```python
from build123d import *

# Parameters (mm, degrees)
F2_DEPTH = 2.5
F3_R     = 3
F4_R     = 20


with BuildPart() as f2:
    # F1 (on Top) → F2 (new body)
    with BuildSketch(Plane.XY):
        with BuildLine():
            Line((2.488848, -10.5), (-2.488848, -10.5))
            Line((-2.488848, -10.5), (-2.488848, -9.168186))
            ThreePointArc((-2.488848, -9.168186), (-4.247392, -2.645334), (-8.899342, 2.253587))
            Line((-8.899342, 2.253587), (-8.899342, 6.253587))
            Line((-8.899342, 6.253587), (-15, 6.253587))
            Line((-15, 6.253587), (-10, -23.746413))
            Line((-10, -23.746413), (-10, -83.746413))
            ThreePointArc((-10, -83.746413), (0, -93.746413), (10, -83.746413))
            Line((10, -83.746413), (10, -23.746413))
            Line((10, -23.746413), (15, 6.253587))
            Line((15, 6.253587), (8.899342, 6.253587))
            Line((8.899342, 6.253587), (8.899342, 2.253587))
            ThreePointArc((8.899342, 2.253587), (4.247392, -2.645334), (2.488848, -9.168186))
            Line((2.488848, -9.168186), (2.488848, -10.5))
        make_face()
    extrude(amount=F2_DEPTH)

    # F3
    f3_edges = [f2.edges().sort_by_distance(p)[0] for p in [
        (-15, 6.253587, 1.25),
        (15, 6.253587, 1.25),
    ]]
    fillet(f3_edges, radius=F3_R)

    # F4
    f4_edges = [f2.edges().sort_by_distance(p)[0] for p in [
        (-10, -23.746413, 1.25),
        (10, -23.746413, 1.25),
    ]]
    fillet(f4_edges, radius=F4_R)


solid = f2.part
```
Verification items for the finished model (mm, model axes). A direction names the side the tool comes from. Coordinates: 2 decimals unless noted, no trailing zeros. Order: outer loops, then holes, each group sorted by start corner. A loop starts at its lowest first (then second) coordinate and runs counter-clockwise, first axis right, second up. Notation, with made-up numbers: (54.25, -28) -> (94.25, -28) arc R22 ccw to (94.25, 10) -> close; hole circle Ø10 at (0.25, 2). An arc over 180 degrees is marked (long way). Answer as CSV lines item,"result". Start each with the question number.
1) Material ranges on L1, parallel to X at y = -59.5, z = 2.35; L2, parallel to Y at x = 0, z = 0.25; L3, parallel to Y at x = 8.5, z = 0.8, recorded low to high. Write a range as [from, to].
2) Set-up check for faces 1 (the face through (-10, 6.254, 1)), 2 (the face through (10, -55, 1)), 3 (the face through (0, -43, 0)), 4 (the face through (-4.2, -2.73, 1.23)), 5 (the face through (-10, -54, 1)): record each of +Z, -Z, +X, -X, +Y, -Y from which the full face is reachable in a straight line by a thin tool's end or side.
3) Cross-section at A-A, the plane z = 1.3. Record the boundary of the cut face in (x, y), then the cut area to 3 significant figures.
4) Gauge pin test, flat ends, axial feed: pin 1 Ø0.8 at (y, z) = (-51, 0.5) entering from -X; pin 2 Ø0.8 at (y, z) = (-56.5, 1) entering from +X; pin 3 Ø1.5 at (y, z) = (-10, 1.5) entering from +X. Record the tip position at first contact, or that the pin passes through.
5) Cross-section at B-B, the plane y = -4. Record the boundary of the cut face in (x, z), then the cut area to 3 significant figures.
6) Release check for a two-part mould opening along X. For faces 6 (the face through (0, -43, 2.5)), 7 (the face through (-0.22, -93.744, 1.232)), 8 (the face through (-8.899, 4, 1)), 9 (the face through (0, -10.5, 1)) record: released by +X, released by -X, zero draft, split by the parting line, or undercut.
7) Cross-section at D-D, the plane x = 0. Record the boundary of the cut face in (y, z).
8) Cross-section at C-C, the plane y = -68.5. Record the boundary of the cut face in (x, z), then the cut area to 3 significant figures.
Conclusion:
1,L1,"x = [-10, 10]"
1,L2,"y = [-93.75, -10.5]"
1,L3,"y = [-89.01, 1.99]"
2,face 1,"+Z, -Z, +X, -X, +Y"
2,face 2,"+Z, -Z, +X, -Y"
2,face 3,"-Z, +X, -X, +Y, -Y"
2,face 4,"+Z, -Z, +Y"
2,face 5,"+Z, -Z, -X, -Y"
3,outline,"(-14.42, 2.76) -> (-10.27, -22.11) arc R20 cw to (-10, -25.4) -> (-10, -83.75) arc R10 ccw to (10, -83.75) -> (10, -25.4) arc R20 cw to (10.27, -22.11) -> (14.42, 2.76) arc R3 ccw to (11.46, 6.25) -> (8.9, 6.25) -> (8.9, 2.25) arc R13.76 ccw to (2.49, -9.17) -> (2.49, -10.5) -> (-2.49, -10.5) -> (-2.49, -9.17) arc R13.76 ccw to (-8.9, 2.25) -> (-8.9, 6.25) -> (-11.46, 6.25) arc R3 ccw to start"
3,area,"1,920 mm²"
4,pin 1,"stops at x = -10"
4,pin 2,"stops at x = 10"
4,pin 3,"stops at x = 12.42"
5,outline,"(-13.29, 0) -> (-3.58, 0) -> (-3.58, 2.5) -> (-13.29, 2.5) -> close; (3.58, 0) -> (13.29, 0) -> (13.29, 2.5) -> (3.58, 2.5) -> close"
5,area,"48.5 mm²"
6,face 6,"zero draft"
6,face 7,"split by the parting line"
6,face 8,"undercut"
6,face 9,"undercut"
7,outline,"(-93.75, 0) -> (-10.5, 0) -> (-10.5, 2.5) -> (-93.75, 2.5) -> close"
8,outline,"(-10, 0) -> (10, 0) -> (10, 2.5) -> (-10, 2.5) -> close"
8,area,"50.0 mm²"
